Autodesk Inventor part; units mm, degrees
ref_plane "YZ Plane" through (0, 0, 0) normal (1, 0, 0) x (0, 1, 0)
ref_plane "XZ Plane" through (0, 0, 0) normal (0, 1, 0) x (-1, 0, 0)
ref_plane "XY Plane" through (0, 0, 0) normal (0, 0, 1) x (1, 0, 0)
sketch "スケッチ1" plane through (0, 0, 0) normal (0, 0, 1) x (1, 0, 0)
  line L0 (0, 0) -> (0, 6.25) construction
  line L1 (0, 6.25) -> (-10, 6.25)
  line L2 (-10, 6.25) -> (-10, 17)
  line L3 (-10, 17) -> (0, 17)
  line L4 (0, 6.25) -> (10, 6.25)
  line L5 (10, 6.25) -> (10, 17)
  line L6 (10, 17) -> (0, 17)
  line L7 (-14, 0) -> (14, 0)
  dimension "d0" = 6.25
  dimension "d1" = 10
  dimension "d2" = 10.75
revolve "回転1" add sketch "スケッチ1" angle 180 mid plane about axis through (-10, 0, 0) along (1, 0, 0)
sketch "スケッチ2" plane through (-10, 0, 17) normal (0, -1, 0) x (1, 0, 0)
  line L0 (20, 0) -> (0, 0)
  line L1 (20, -10.75) -> (20, 0)
  point P0 (10, -17)
  point P1 (16, -4)
  dimension "d4" = 4
  dimension "d5" = 4
hole "穴1" at (6, 0, 13) direction (0, 1, 0) diameter 3.242 end through all
mirror "ミラー1" about plane through (0, 0, 0) normal (0, 0, 1) of "穴1"
sketch "スケッチ3" plane through (-10, 0, -17) normal (-1, 0, 0) x (0, 0, 1)
  circle A0 centre (17, 0) radius 15.5
  dimension "d16" = 31
extrude "押し出し1" cut sketch "スケッチ3" against normal blind 12
chamfer "面取り2" distance 0.75 angle 45 2 edges at (10, 17, 0) (-10, 17, 0)
properties part number "probe-cover" material "ステンレス鋼"
Verification items for the finished model (mm, model axes). Coordinates: 2 decimals unless noted, no trailing zeros. Write each loop counter-clockwise with the first axis right and the second up, starting at its lowest first coordinate (ties: lowest second). Pieces come first, ordered by that corner, then holes. Notation, with made-up numbers: (40, 81) - (54, 81) arc R23 ccw to (54, 118) - close; hole circle Ø5 at (12.25, 16.5). An arc over 180 degrees is marked (long way). Answer as a JSON object with one key per item and string values.
(1) Cross-section at A-A on x = 6. Record the cut outline in (y, z), plus the area to 3 significant figures.
Report:
{"outline": "(0, -17) arc R17 ccw to (8.67, -14.62) - (0, -14.62) - close; (0, -11.38) - (12.63, -11.38) arc R17 ccw to (12.63, 11.38) - (0, 11.38) - (0, 6.25) arc R6.25 cw to (0, -6.25) - close; (0, 14.62) - (8.67, 14.62) arc R17 ccw to (0, 17) - close", "area": "322 mm^2"}
(2) Thickness scan on line 1 along Z through (x, y) = (6, 7); line 2 along X through (y, z) = (5.25, 13); line 3 along Z through (x, y) = (6, 2.5). Record the ranges inside material, lowest first.
Report:
{"line 1": "-15.49 to -14.62, -11.38 to 11.38, 14.62 to 15.49", "line 2": "2 to 4.38, 7.62 to 10", "line 3": "-16.82 to -14.62, -11.38 to -5.73, 5.73 to 11.38, 14.62 to 16.82"}
(3) Mould release check, pull along Z, two halves, no side actions. Record for faces 1 (the flat face through (2, 8, 0)), 2 (the flat face through (10, 8, 0)), 3 (the conical face through (-9.87, 16.376, -0.36)), 4 (the cylindrical face through (-4.084, 15.496, 0.341)): pulls with the +Z half, pulls with the -Z half, needs draft (parallel to the pull), parting line crosses it, or undercut.
Report:
{"face 1": "undercut", "face 2": "needs draft", "face 3": "parting line crosses it", "face 4": "undercut"}
(4) Cross-section at D-D on y = 7.5. Give the number of separate pieces and of enclosed holes in the cut face, plus the area to 3 significant figures.
Report:
{"separate pieces": "1", "enclosed holes": "2", "area": "267 mm^2"}
(5) Cross-section at B-B on z = 0. Record the cut outline in (x, y), plus the area to 3 significant figures.
Report:
{"outline": "(-10, 15.5) - (2, 15.5) - (2, 6.25) - (10, 6.25) - (10, 16.25) - (9.25, 17) - (-9.25, 17) - (-10, 16.25) - close", "area": "103 mm^2"}
(6) Cross-section at C-C on x = -6. Record the cut outline in (y, z), plus the area to 3 significant figures.
Report:
{"outline": "(0, -17) arc R17 ccw to (0, 17) - (0, 15.5) arc R15.5 cw to (0, -15.5) - close", "area": "76.6 mm^2"}
(7) Gauge pin test, flat ends, axial feed: pin 1 Ø1 at (x, z) = (-3, 8.5) entering from -Y; pin 2 Ø2 at (x, y) = (-1, 2.5) entering from -Z; pin 3 Ø4 at (y, z) = (6.5, -9) entering from -X. Record the tip position at first contact, or that the pin passes through.
Report:
{"pin 1": "y = 12.62", "pin 2": "z = -16.93", "pin 3": "x = 2"}
